Part print with two shaded views. Sizes in mm from the minimum x, y, z corner. Give positions to 0.01 mm unless a question says otherwise; leave off trailing zeros. Write each loop counter-clockwise with the first axis right and the second up, starting at its lowest first coordinate (ties: lowest second). Pieces come first, ordered by that corner, then holes. Notation, with made-up numbers: M 18,33 L 29,33 A17 ccw 29,44 Z; hole C 41,70 d5. An arc over 180 degrees is marked long. Return JSON: item names as keys, results as strings. Group by question number.
Q1. Band-saw the part on A-A, the plane y = 25. Give the cut face in (x, z).
Q2. Band-saw the part on D-D, the plane x = 44. Give the cut face in (y, z), then the cut area to 3 significant figures.
Q3. Flat gauge pins, fed straight in: pin 1 Ø0.9 at (x, z) = (1, 1) entering from -Y; pin 2 Ø5.5 at (x, y) = (48, 25) entering from +Z; pin 3 Ø5 at (x, y) = (18.5, 25) entering from -Z; pin 4 Ø1.5 at (y, z) = (24.5, 2) entering from -X. Where does each tip first touch, or does it go through?
Q4. Wall check: probe 1 along Y at (x, z) = (48, 1); probe 2 along Y at (x, z) = (36.5, 0.2); probe 3 along X at (y, z) = (23.5, 1.3). Give the ranges that are in metal, low to high.
Q5. Band-saw the part on C-C, the plane x = 13.1. Give the cut face in (y, z).
Q6. Band-saw the part on B-B, the plane z = 1. Count the separate pieces of the cut face and the enclosed holes in it, then the cut area to 3 significant figures.
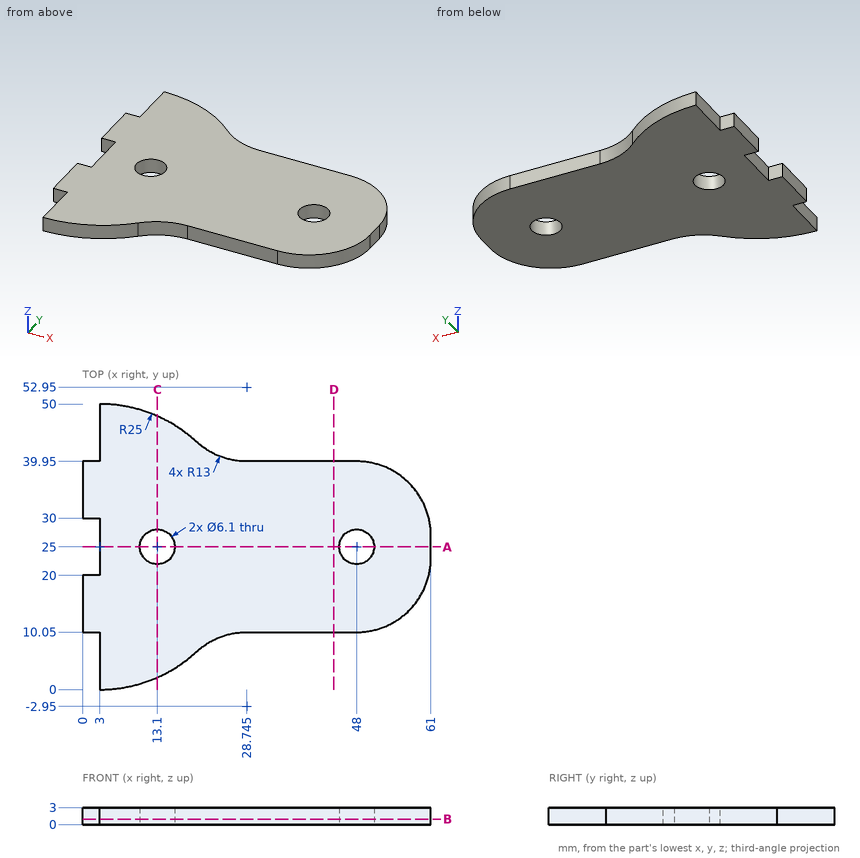
From the geometry:
{
 "1": {"outline": "M 3,0 L 10.05,0 L 10.05,3 L 3,3 Z; M 16.15,0 L 44.95,0 L 44.95,3 L 16.15,3 Z; M 51.05,0 L 61,0 L 61,3 L 51.05,3 Z"},
 "2": {"outline": "M 10.05,0 L 39.95,0 L 39.95,3 L 10.05,3 Z", "area": "89.7 mm^2"},
 "3": {"pin 1": "stops at y = 10.05", "pin 2": "passes through", "pin 3": "stops at z = 0", "pin 4": "stops at x = 3"},
 "4": {"probe 1": "y = 10.05 to 21.95, 28.05 to 39.95", "probe 2": "y = 10.05 to 39.95", "probe 3": "x = 3 to 10.44, 15.76 to 45.34, 50.66 to 61"},
 "5": {"outline": "M 2.13,0 L 21.95,0 L 21.95,3 L 2.13,3 Z; M 28.05,0 L 47.87,0 L 47.87,3 L 28.05,3 Z"},
 "6": {"separate pieces": "1", "enclosed holes": "2", "area": "1,950 mm^2"}
}
